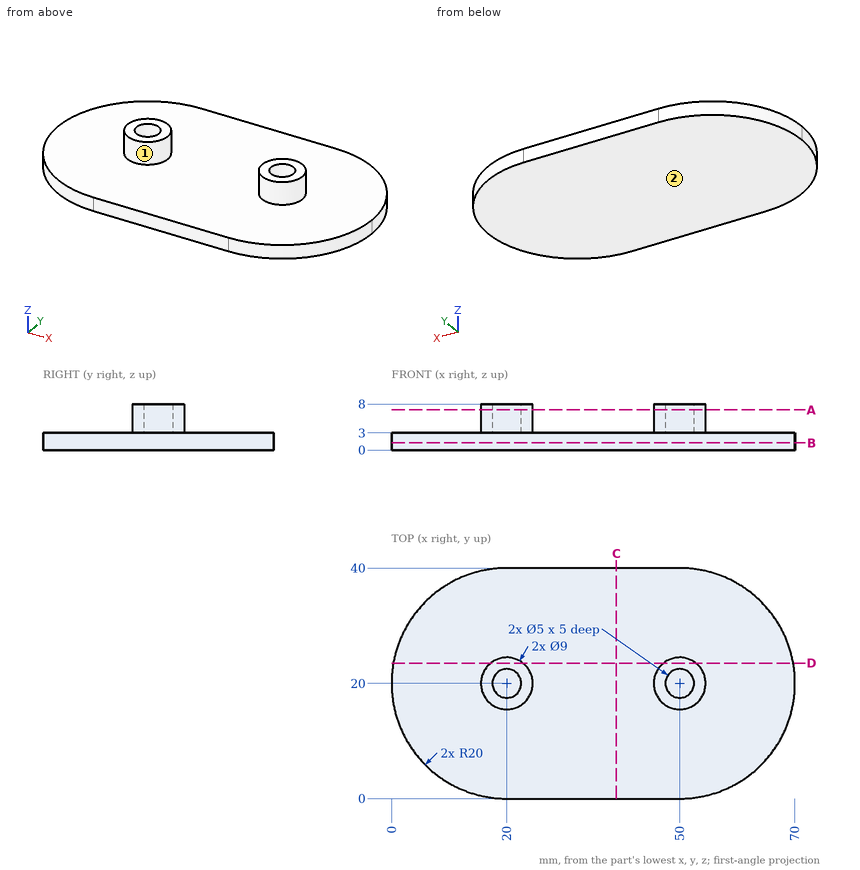
Geometry check sheet. Reference: drawing and pictorial views, mm from the part's lowest x, y, z. Coordinates: 2 decimals unless noted, no trailing zeros. Order: outer loops, then holes, each group sorted by start corner. A loop starts at its lowest first (then second) coordinate and runs counter-clockwise, first axis right, second up.
Item 1: Depth check by flat-ended pin: pin 1 (8 mm diameter, centred on x = 15.5, y = 33, fed in from -Z). Enter the tip coordinate at first touch or a pass-through.
Item 2: Mould release check, pull along X, two halves, no side actions. Record for the marked faces 1 and 2: released by +X, released by -X, zero draft, split by the parting line, or undercut.
Item 3: Section check A-A (z = 7). Enter the section's corners in (x, y).
Item 4: Section check C-C (x = 39). Enter the section's corners in (y, z).
Item 5: Section check B-B (z = 1.25). Enter the section's corners in (x, y), plus the area to 3 significant figures.
Item 6: Scan lines: line 1 along Y through (x, z) = (20, 5.7); line 2 along Z through (x, y) = (37, 13); line 3 along Y through (x, z) = (15.5, 1.25). Record each from-to range of solid material in increasing order.
Item 7: Section check D-D (y = 23.5). Enter the section's corners in (x, z).
Check sheet entries:
1. pin 1: stops at z = 0
2. face 1: undercut
2. face 2: zero draft
3. outline: circle Ø9 at (20, 20); circle Ø9 at (50, 20); hole circle Ø5 at (20, 20); hole circle Ø5 at (50, 20)
4. outline: (0, 0) - (40, 0) - (40, 3) - (0, 3) - close
5. outline: (0, 20) arc R20 ccw to (20, 0) - (50, 0) arc R20 ccw to (70, 20) arc R20 ccw to (50, 40) - (20, 40) arc R20 ccw to start
5. area: 2,460 mm2
6. line 1: y = 15.5 to 17.5, 22.5 to 24.5
6. line 2: z = 0 to 3
6. line 3: y = 0.51 to 39.49
7. outline: (0.31, 0) - (69.69, 0) - (69.69, 3) - (52.83, 3) - (52.83, 8) - (47.17, 8) - (47.17, 3) - (22.83, 3) - (22.83, 8) - (17.17, 8) - (17.17, 3) - (0.31, 3) - close
